from build123d import *

# Parameters (mm, degrees)
F2_R            = 9.9
F3_DEPTH        = 25
F5_DEPTH        = 25
F5_COPIES_COUNT = 23
F7_R            = 2.95
F8_DEPTH        = 37.3


# Not quite as in the source:
# - a feature of the source that left no trace in its solid (it failed there, or was rolled back) is left out
# - a pattern or mirror of a feature is missing from the dataset's text; its kind, count and spacing are read off the source's solid


with BuildPart() as f1:
    # F0 (on Right) → F1 (revolve)
    with BuildSketch(Plane.YZ):
        Polygon((0, 24.65), (0, 0), (20.2, 0), (20.2, 15.95), (10, 15.95), (10, 24.65), align=None)
    revolve(axis=Axis((0, 10.1, 0), (0, 1, 0)))

    # F2 (on face) → F3 (cut)
    with BuildSketch(Plane(origin=(0, 20.2, 0), x_dir=(-1, 0, 0), z_dir=(0, 1, 0))):
        Circle(F2_R)
    extrude(amount=-F3_DEPTH, mode=Mode.SUBTRACT)

    # F4 (on face) → F5 (cut)
    with BuildSketch(Plane.XZ):
        with BuildLine():
            ThreePointArc((0.9605272399, 20.4764837905), (1.5385061373, 22.5929437067), (2.6011700561, 24.5123726787))
            ThreePointArc((2.6011700561, 24.5123726787), (0, 24.65), (-2.6011700561, 24.5123726787))
            ThreePointArc((-2.6011700561, 24.5123726787), (-1.5385061373, 22.5929437067), (-0.9605272399, 20.4764837905))
            ThreePointArc((-0.9605272399, 20.4764837905), (0, 20.499), (0.9605272399, 20.4764837905))
        make_face()
        with BuildLine():
            ThreePointArc((2.6011700561, 24.5123726787), (2.8144449637, 24.7961797548), (3.0385106282, 25.0715471833))
            ThreePointArc((3.0385106282, 25.0715471833), (0, 25.255), (-3.0385106282, 25.0715471833))
            ThreePointArc((-3.0385106282, 25.0715471833), (-2.8144449637, 24.7961797548), (-2.6011700561, 24.5123726787))
            ThreePointArc((-2.6011700561, 24.5123726787), (0, 24.65), (2.6011700561, 24.5123726787))
        make_face()
    f5 = extrude(amount=-F5_DEPTH, mode=Mode.SUBTRACT)

    # F5_copies: F5 ×23 about axis
    f5_copies_axis = Axis((0, 0, 0), (0, 1, 0))
    for i in range(1, F5_COPIES_COUNT):
        add(f5.rotate(f5_copies_axis, i * 360 / F5_COPIES_COUNT), mode=Mode.SUBTRACT)

    # F7 (on Right) → F8 (cut, symmetric)
    with BuildSketch(Plane.YZ):
        with Locations((15.15, 1.0436970042)):
            Circle(F7_R)
    extrude(amount=F8_DEPTH, both=True, mode=Mode.SUBTRACT)


solid = f1.part
Geometry: final body of the model. Coordinates: model frame, mm. A direction names the side the tool comes from. Coordinates: 2 decimals unless noted, no trailing zeros. Order: outer loops, then holes, each group sorted by start corner. A loop starts at its lowest first (then second) coordinate and runs counter-clockwise, first axis right, second up.
(1) Access query for faces 1 (the face through (-22.616, 4.93, -0.016)), 2 (the face through (13.056, 4.93, -18.467)), 3 (the face through (-23.23, 4.93, 8.24)), 4 (the face through (-10.4, 20.2, 0.2)), 5 (the face through (-1.55, 4.93, 22.62)). Directions: +Z, -Z, +X, -X, +Y, -Y. A direction counts if a zero-diameter tool reaches every point of the face in a straight line with its end or side. Return the directions, or none.
(2) Draft query along Z for faces 6 (the face through (-12.45, 16.74, 3.53)), 7 (the face through (23.223, 4.93, 8.265)), 8 (the face through (12.95, 4.93, -15.89)), 9 (the face through (10.4, 4.9, -20.1)). Return one class per face: pulls with the +Z half, pulls with the -Z half, needs draft (parallel to the pull), parting line crosses it, or undercut.
(3) Material intervals for probe 1 along Z at (x, y) = (12.5, 15.15); probe 2 along Y at (x, z) = (19.5, 2); probe 3 along Z at (x, y) = (-13.5, 15.15), sorted ascending.
(4) First-contact query: pin 1 (6 mm diameter, centred on x = -11, y = 11.5, fed in from -Z); pin 2 (2 mm diameter, centred on x = 15.5, y = 5, fed in from -Z); pin 3 (10 mm diameter, centred on x = -8, y = 8, fed in from +Z); pin 4 (5.5 mm diameter, centred on y = 15.15, z = 1.04, fed in from -X). Flat tips, straight axial feed; report the tip coordinate or a pass-through.
(5) Section query B-B (y = 15.15). Return the cut outline in (x, z), plus the area to 3 significant figures.
(6) Section query A-A (x = 0). Return the cut outline in (y, z), plus the area to 3 significant figures.
Solution:
1. face 1: -X, +Y, -Y
1. face 2: +Y, -Y
1. face 3: +Z, -X, +Y, -Y
1. face 4: +Z, -Z, +X, -X, +Y
1. face 5: +Z, +Y, -Y
2. face 6: undercut
2. face 7: pulls with the +Z half
2. face 8: undercut
2. face 9: pulls with the -Z half
3. probe 1: z = -9.91 to -1.91, 3.99 to 9.91
3. probe 2: y = 0 to 10
3. probe 3: z = -8.49 to -1.91, 3.99 to 8.49
4. pin 1: stops at z = -21.45
4. pin 2: stops at z = -17.05
4. pin 3: stops at z = 24.47
4. pin 4: passes through
5. outline: (-15.84, -1.91) arc R15.95 ccw to (15.84, -1.91) - (9.71, -1.91) arc R9.9 cw to (-9.71, -1.91) - close; (-15.44, 3.99) - (-9.06, 3.99) arc R9.9 cw to (9.06, 3.99) - (15.44, 3.99) arc R15.95 ccw to start
5. area: 419 mm2
6. outline: (0, -24.65) - (10, -24.65) - (10, -15.95) - (20.2, -15.95) - (20.2, -9.9) - (0, -9.9) - close; (0, 9.9) - (20.2, 9.9) - (20.2, 15.95) - (10, 15.95) - (10, 20.5) - (0, 20.5) - close
6. area: 377 mm2
